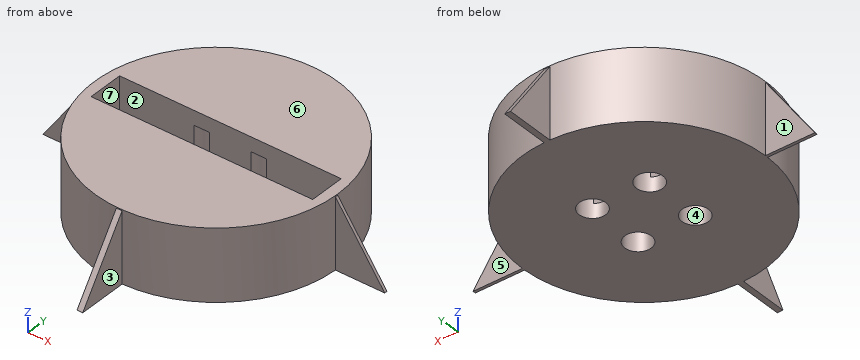
from build123d import *

# Parameters (mm, degrees)
F0_R      = 85
F1_DEPTH  = 50
F2_R      = 9.25
F3_DEPTH  = 40
F4_W      = 155
F4_H      = 25
F5_DEPTH  = 40
F7_DEPTH  = 2
F10_DEPTH = 2


with BuildPart() as f1:
    # F0 (on Top) → F1 (new body)
    with BuildSketch(Plane.XY):
        Circle(F0_R)
    extrude(amount=F1_DEPTH)

    # F2 (on face) → F3 (cut)
    with BuildSketch(Plane(origin=(0, 0, 0), x_dir=(1, 0, 0), z_dir=(0, 0, -1))):
        with Locations((20, 20)):
            Circle(F2_R)
        with Locations((-20, 20)):
            Circle(F2_R)
        with Locations((-20, -20)):
            Circle(F2_R)
        with Locations((20, -20)):
            Circle(F2_R)
    extrude(amount=-F3_DEPTH, mode=Mode.SUBTRACT)

    # F4 (on face) → F5 (cut)
    with BuildSketch(Plane.XY.offset(50)):
        Rectangle(F4_W, F4_H)
    extrude(amount=-F5_DEPTH, mode=Mode.SUBTRACT)

    # F6 (on Right) → F7 (join)
    with BuildSketch(Plane.YZ):
        Polygon((-119.5, 0), (-84.5, 0), (-84.5, 50), align=None)
    extrude(amount=F7_DEPTH)

    # F8: F1 across plane


with BuildPart() as f1_1:
    add(f1.part)
    add(f1.part.mirror(Plane.XZ))

    # F9 (on Front) → F10 (join)
    with BuildSketch(Plane.XZ):
        Polygon((-84.5, 0), (-84.5, 50), (-119.5, 0), align=None)
    extrude(amount=F10_DEPTH)

    # F11: F1 across plane


with BuildPart() as f1_2:
    add(f1_1.part)
    add(f1_1.part.mirror(Plane.YZ))


solid = f1_2.part
The listing builds one solid part. Answer for the finished solid, in the listing's coordinates (mm). Face numbers are marked on the shaded views. A direction names the side the tool comes from. Give positions to 0.01 mm unless a question says otherwise; leave off trailing zeros. Loops run counter-clockwise (first coordinate to the right, second up) from the corner with the lowest first, then second, coordinate; pieces in that order, holes last.
Item 1: Determine the mould class of the marked faces 5, 6 and 7 for opening direction Y: +Y half, -Y half, draft (parallel to the pull), parting line (faces both ways), or undercut.
Derived:
face 5: +Y half
face 6: draft
face 7: undercut
Item 2: A cutting plane is placed at C-C (z = 28.5). Give the vertices of the cut face in (x, y), then the cut area to 3 significant figures.
Derived:
outline: (-99.55, -2) - (-84.98, -2) arc R85 ccw to (-2, -84.98) - (-2, -99.55) - (2, -99.55) - (2, -84.98) arc R85 ccw to (84.98, -2) - (99.55, -2) - (99.55, 0) - (85, 0) arc R85 ccw to (2, 84.98) - (2, 99.55) - (-2, 99.55) - (-2, 84.98) arc R85 ccw to (-85, 0) - (-99.55, 0) - close; hole (-77.5, -12.5) - (-25.41, -12.5) arc R9.25 ccw (long way) to (-14.59, -12.5) - (14.59, -12.5) arc R9.25 ccw (long way) to (25.41, -12.5) - (77.5, -12.5) - (77.5, 12.5) - (25.41, 12.5) arc R9.25 ccw (long way) to (14.59, 12.5) - (-14.59, 12.5) arc R9.25 ccw (long way) to (-25.41, 12.5) - (-77.5, 12.5) - close
area: 18,000 mm2
Item 3: Find the intervals of material crossed by line 1 along X through (y, z) = (20, 17); line 2 along Y through (x, z) = (-13.5, 12); line 3 along Y through (x, z) = (-65, 31), in increasing order.
Derived:
line 1: x = -82.61 to -29.25, -10.75 to 10.75, 29.25 to 82.61
line 2: y = -83.92 to -26.58, -13.42 to -12.5, 12.5 to 13.42, 26.58 to 83.92
line 3: y = -54.77 to -12.5, 12.5 to 54.77
Item 4: A cutting plane is placed at A-A (z = 3). Give the vertices of the cut face in (x, y).
Derived:
outline: (-117.4, -2) - (-84.98, -2) arc R85 ccw to (-2, -84.98) - (-2, -117.4) - (2, -117.4) - (2, -84.98) arc R85 ccw to (84.98, -2) - (117.4, -2) - (117.4, 0) - (85, 0) arc R85 ccw to (2, 84.98) - (2, 117.4) - (-2, 117.4) - (-2, 84.98) arc R85 ccw to (-85, 0) - (-117.4, 0) - close; hole circle Ø18.5 at (-20, -20); hole circle Ø18.5 at (-20, 20); hole circle Ø18.5 at (20, -20); hole circle Ø18.5 at (20, 20)
Item 5: A cutting plane is placed at D-D (y = -20). Give the vertices of the cut face in (x, z).
Derived:
outline: (-82.61, 0) - (-29.25, 0) - (-29.25, 40) - (-10.75, 40) - (-10.75, 0) - (10.75, 0) - (10.75, 40) - (29.25, 40) - (29.25, 0) - (82.61, 0) - (82.61, 50) - (-82.61, 50) - close
Item 6: A tool of negligible diameter and unlimited length cuts with its end or side. For the marked faces 1, 2, 3 and 4, from which of +Z, -Z, +X, -X, +Y, -Y can it reach the whole face along a straight path? Write none if from no direction.
Derived:
face 1: +Z, -Z, -X, +Y
face 2: +Z
face 3: +Z, -Z, +X, -Y
face 4: -Z
Item 7: A cutting plane is placed at B-B (x = 20). Give the vertices of the cut face in (y, z), then the cut area to 3 significant figures.
Derived:
outline: (-82.61, 0) - (-29.25, 0) - (-29.25, 40) - (-12.5, 40) - (-12.5, 50) - (-82.61, 50) - close; (-10.75, 0) - (10.75, 0) - (10.75, 10) - (-10.75, 10) - close; (12.5, 40) - (29.25, 40) - (29.25, 0) - (82.61, 0) - (82.61, 50) - (12.5, 50) - close
area: 5,890 mm2
Item 8: Each of these flat-tipped pins is pushed along its axis until it touches: pin 1 Ø15 at (x, y) = (-20, -20) entering from -Z; pin 2 Ø4 at (y, z) = (60, 18.5) entering from -X; pin 3 Ø17.5 at (x, z) = (108.5, 18) entering from -Y; pin 4 Ø8 at (x, y) = (-23, 89.5) entering from +Z (3 decimals). Where does it stop, or does it pass through?
Derived:
pin 1: stops at z = 40
pin 2: stops at x = -62.14
pin 3: stops at y = -2
pin 4: passes through
